The model under review builds one solid part; all positions refer to its coordinate system, in mm. Coordinates: 2 decimals unless noted, no trailing zeros. Order: outer loops, then holes, each group sorted by start corner. A loop starts at its lowest first (then second) coordinate and runs counter-clockwise, first axis right, second up. Notation, with made-up numbers: (14.5, 36) - (52.5, 36) arc R24 ccw to (52.5, 60) - close; hole circle Ø1 at (-16, 51). An arc over 180 degrees is marked (long way). Answer in a Markdown table with one row per item.
```python
from build123d import *

# Parameters (mm, degrees)
SKETCH1_W           = 168.412
SKETCH1_H           = 15
BOSS_EXTRUDE1_DEPTH = 5.588
SKETCH2_R           = 1.75
CUT_EXTRUDE1_DEPTH  = 98.959199068
SKETCH3_R           = 1.75
CUT_EXTRUDE2_DEPTH  = 98.959199068


with BuildPart() as part:
    # Sketch1 → Boss-Extrude1 (new body)
    with BuildSketch(Plane(origin=(0, 0, 0), x_dir=(1, 0, 0), z_dir=(0, 1, 0))):
        with Locations((12.851084959, 4.52918108)):
            Rectangle(SKETCH1_W, SKETCH1_H)
    extrude(amount=BOSS_EXTRUDE1_DEPTH)

    # Sketch2 → Cut-Extrude1 (cut, through all)
    with BuildSketch(Plane(origin=(0, 5.588, 0), x_dir=(1, 0, 0), z_dir=(0, 1, 0))):
        with Locations(Location((-59.354915041, 4.52918108, 0), (0, 0, 270))):
            Circle(SKETCH2_R)
        with Locations(Location((-49.354915041, 4.52918108, 0), (0, 0, 270))):
            Circle(SKETCH2_R)
        with Locations(Location((75.057084959, 4.52918108, 0), (0, 0, 270))):
            Circle(SKETCH2_R)
        with Locations(Location((85.057084959, 4.52918108, 0), (0, 0, 270))):
            Circle(SKETCH2_R)
    extrude(amount=-CUT_EXTRUDE1_DEPTH, mode=Mode.SUBTRACT)

    # Sketch3 → Cut-Extrude2 (cut, through all)
    with BuildSketch(Plane(origin=(0, 5.588, 0), x_dir=(1, 0, 0), z_dir=(0, 1, 0))):
        with Locations(Location((-4.648915041, 4.52918108, 0), (0, 0, 270))):
            Circle(SKETCH3_R)
        with Locations(Location((30.351084959, 4.52918108, 0), (0, 0, 270))):
            Circle(SKETCH3_R)
        with Locations(Location((12.851084959, 4.52918108, 0), (0, 0, 270))):
            Circle(SKETCH3_R)
    extrude(amount=-CUT_EXTRUDE2_DEPTH, mode=Mode.SUBTRACT)


solid = part.part
```
Item 1: We need section A-A, the plane z = -4.75. State how many separate pieces and enclosed holes the cut face has, then the cut area to 3 significant figures.
Check values:
| item | result |
|---|---|
| separate pieces | 8 |
| enclosed holes | 0 |
| area | 805 mm^2 |
Item 2: We need section B-B, the plane y = 3.6. Write out the cut boundary in (x, z).
Check values:
| item | result |
|---|---|
| outline | (-71.35, -12.03) - (97.06, -12.03) - (97.06, 2.97) - (-71.35, 2.97) - close; hole circle Ø3.5 at (-59.35, -4.53); hole circle Ø3.5 at (-49.35, -4.53); hole circle Ø3.5 at (-4.65, -4.53); hole circle Ø3.5 at (12.85, -4.53); hole circle Ø3.5 at (30.35, -4.53); hole circle Ø3.5 at (75.06, -4.53); hole circle Ø3.5 at (85.06, -4.53) |
Item 3: To check wall thickness, follow line 1 (Z direction, x = 75, y = 2.85); line 2 (Z direction, x = -60.5, y = 5.15). State the ranges of each line that lie inside material, in increasing order. Write a range as from..to.
Check values:
| item | result |
|---|---|
| line 1 | -12.03..-6.28, -2.78..2.97 |
| line 2 | -12.03..-5.85, -3.21..2.97 |
Item 4: Mouldability with a two-part tool opening along Z and no side actions: class faces 1 (the face through (-51.063, 2.833, -4.909)), 2 (the face through (97.057, 3, -4)), 3 (the face through (12, 3, -12.029)) as +Z half, -Z half, draft (parallel to the pull), parting line (faces both ways), or undercut.
Check values:
| item | result |
|---|---|
| face 1 | undercut |
| face 2 | draft |
| face 3 | -Z half |
